Could you check a few things on this drawing? It's one solid part, dimensions in mm from its lowest x, y, z. Round coordinates to 2 decimals unless told otherwise and drop trailing zeros. Loops run counter-clockwise (first coordinate to the right, second up) from the corner with the lowest first, then second, coordinate; pieces in that order, holes last. Notation, with made-up numbers: M 76,49.5 L 80,49.5 A37 cw 80,86.5 Z; hole C 67.5,51.5 d10. An arc over 180 degrees is marked long. Answer as a JSON object with one key per item and string values.
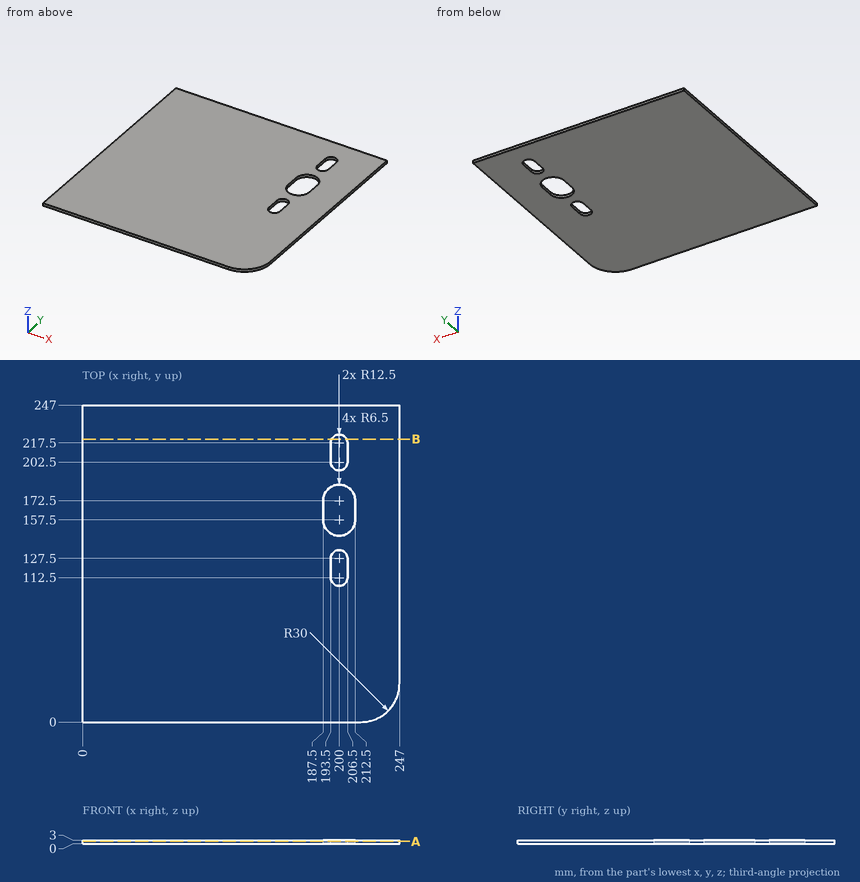
Item 1: I want a section at B-B, the plane y = 220.5. Please give me the cut outline in (x, z).
Resolved:
{"outline": "M 0,0 L 194.23,0 L 194.23,3 L 0,3 Z; M 205.77,0 L 247,0 L 247,3 L 205.77,3 Z"}
Item 2: I want a section at A-A, the plane z = 1.85. Please give me the cut outline in (x, y).
Resolved:
{"outline": "M 0,0 L 217,0 A30 ccw 247,30 L 247,247 L 0,247 Z; hole M 187.5,157.5 A12.5 ccw 212.5,157.5 L 212.5,172.5 A12.5 ccw 187.5,172.5 Z; hole M 193.5,112.5 A6.5 ccw 206.5,112.5 L 206.5,127.5 A6.5 ccw 193.5,127.5 Z; hole M 193.5,202.5 A6.5 ccw 206.5,202.5 L 206.5,217.5 A6.5 ccw 193.5,217.5 Z"}
Item 3: Please list where these lines run through material, in increasing order: probe 1 along X at (y, z) = (202, 0.55); probe 2 along Y at (x, z) = (201.5, 2.05); probe 3 along Y at (x, z) = (218.5, 0.7). Write a range as from..to.
Resolved:
{"probe 1": "0..193.52, 206.48..247", "probe 2": "0..106.18, 133.82..145.09, 184.91..196.18, 223.82..247", "probe 3": "0.04..247"}
